Geometry: see drawing. Coordinates: mm, zero at the bounding-box minimum. A direction names the side the tool comes from. Coordinates: 2 decimals unless noted, no trailing zeros. Write each loop counter-clockwise with the first axis right and the second up, starting at its lowest first coordinate (ties: lowest second). Pieces come first, ordered by that corner, then holes. Notation, with made-up numbers: (51.25, 0) -> (107.25, 0) arc R10 cw to (107.25, 18) -> close; hole circle Ø2 at (-11.75, -39.5). An arc over 180 degrees is marked (long way). Use one line per item in the form item = value. Start each with the question number.
(1) Cut plane C-C on x = 48.5. Return the cut outline in (y, z) (3 decimals), plus the area to 3 significant figures.
(2) First-contact query: pin 1 (15 mm diameter, centred on y = 41, z = 25.5, fed in from -X); pin 2 (1.5 mm diameter, centred on x = 44.5, z = 45, fed in from +Y) (3 decimals). Flat tips, straight axial feed; report the tip coordinate or a pass-through.
(3) Cut plane B-B on y = 29. Return the cut outline in (x, z) (3 decimals).
(4) Set-up query: the marked faces 1 and 2. Return all of +Z, -Z, +X, -X, +Y, -Y with unobstructed straight access to the full face (end or side cutting, diameter ignored); none if empty.
(5) Ray query, line 1 along X through (y, z) = (34, 4) (3 decimals); line 2 along Y through (x, z) = (16.5, 20.5) (3 decimals). Return the intervals inside material, ascending.
(6) Cut plane A-A on z = 13.5. Return the cut outline in (x, y) (3 decimals).
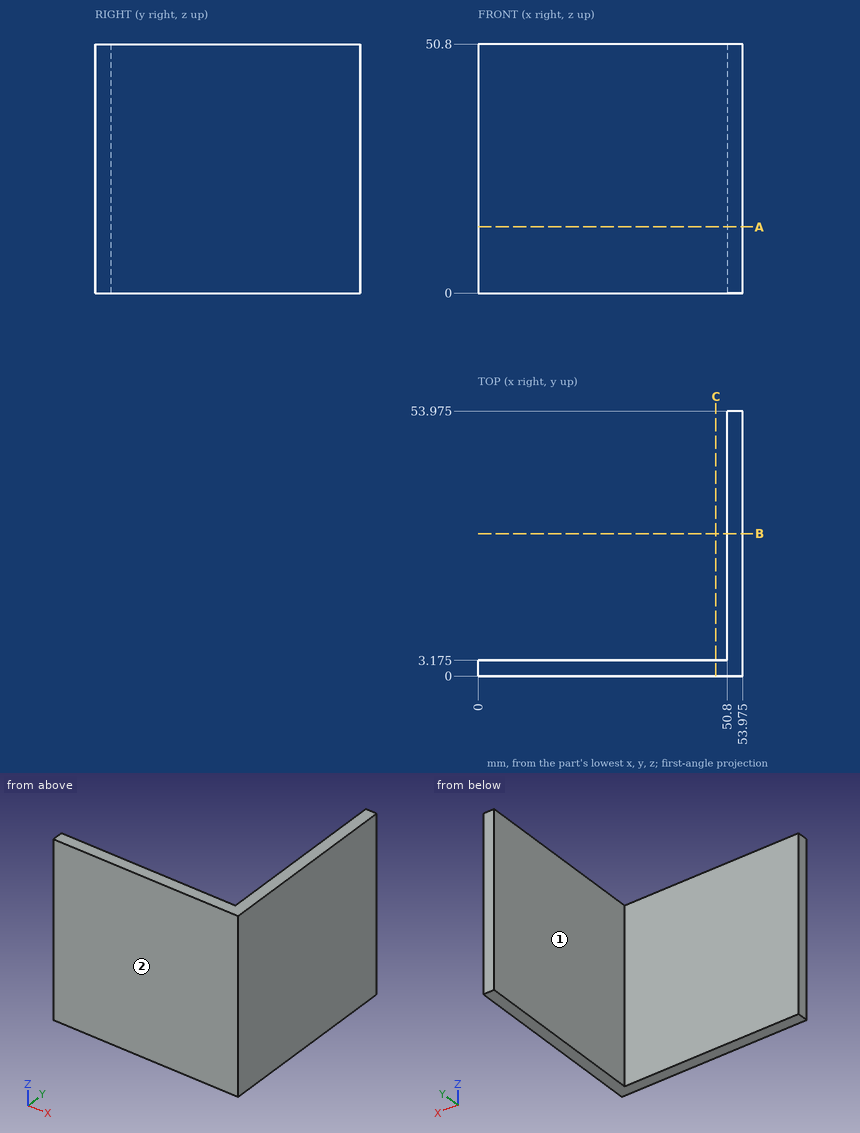
Values:
q1.outline = (0, 0) -> (3.175, 0) -> (3.175, 50.8) -> (0, 50.8) -> close
q1.area = 161 mm2
q2.pin_1 = 50.8
q2.pin_2 = 3.175
q3.outline = (50.8, 0) -> (53.975, 0) -> (53.975, 50.8) -> (50.8, 50.8) -> close
q4.face_1 = +Z, -Z, -X, +Y
q4.face_2 = +Z, -Z, +X, -X, -Y
q5.line_1 = 50.8 to 53.975
q5.line_2 = 0 to 3.175
q6.outline = (0, 0) -> (53.975, 0) -> (53.975, 53.975) -> (50.8, 53.975) -> (50.8, 3.175) -> (0, 3.175) -> close
